The model under review builds one solid part; all positions refer to its coordinate system, in mm. Face numbers are marked on the shaded views. A direction names the side the tool comes from. Give positions to 0.01 mm unless a question says otherwise; leave off trailing zeros. Loops run counter-clockwise (first coordinate to the right, second up) from the corner with the lowest first, then second, coordinate; pieces in that order, holes last. Notation, with made-up numbers: M 14,84 L 33,84 A23 ccw 33,116 Z; hole C 85,25 d10. An arc over 180 degrees is marked long. Return JSON: item names as keys, results as strings.
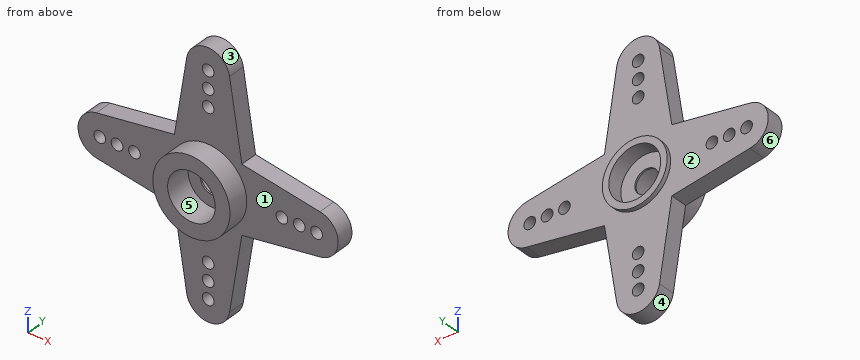
Autodesk Inventor part; units mm, degrees
ref_plane "YZ Plane" through (0, 0, 0) normal (1, 0, 0) x (0, 1, 0)
ref_plane "XZ Plane" through (0, 0, 0) normal (0, 1, 0) x (-1, 0, 0)
ref_plane "XY Plane" through (0, 0, 0) normal (0, 0, 1) x (1, 0, 0)
sketch "Sketch1" plane through (0, 0, 0) normal (0, 1, 0) x (-1, 0, 0)
  circle A0 centre (0, 0) radius 10.5 construction
  circle A1 centre (0, 0) radius 12.5 construction
  circle A2 centre (0, 0) radius 8.5 construction
  circle A3 centre (12.5, 0) radius 2.5
  circle A4 centre (12.5, 0) radius 0.675
  circle A5 centre (10.5, 0) radius 0.675
  circle A6 centre (8.5, 0) radius 0.675
  line L0 (0, 16.4462) -> (0, -19.2601)
  circle A7 centre (0, 12.5) radius 0.675
  circle A8 centre (0, 10.5) radius 0.675
  circle A9 centre (0, 12.5) radius 2.5
  circle A10 centre (0, 8.5) radius 0.675
  circle A11 centre (-12.5, 0) radius 0.675
  circle A12 centre (-10.5, 0) radius 0.675
  circle A13 centre (-12.5, 0) radius 2.5
  circle A14 centre (-8.5, 0) radius 0.675
  circle A15 centre (0, -12.5) radius 0.675
  circle A16 centre (0, -10.5) radius 0.675
  circle A17 centre (0, -12.5) radius 2.5
  circle A18 centre (0, -8.5) radius 0.675
  line L1 (0, 0) -> (7.0711, -7.0711) construction
  line L2 (0, 0) -> (10, 0) construction
  line L3 (0, 0) -> (7.0711, 7.0711) construction
  line L4 (0, 0) -> (10, 0) construction
  line L5 (0, 0) -> (7.0711, -7.0711) construction
  line L6 (0, 0) -> (10, 0) construction
  line L7 (0, 0) -> (-7.0711, -7.0711) construction
  line L8 (0, 0) -> (10, 0) construction
  line L9 (3.8872, -3.8872) -> (12.8889, -2.4696)
  line L10 (3.8872, -3.8872) -> (2.4696, -12.8889)
  line L11 (3.8872, 3.8872) -> (2.4696, 12.8889)
  line L12 (3.8872, 3.8872) -> (12.8889, 2.4696)
  line L13 (-3.8872, 3.8872) -> (-12.8889, 2.4696)
  line L14 (-3.8872, 3.8872) -> (-2.4696, 12.8889)
  line L15 (-3.8872, -3.8872) -> (-2.4696, -12.8889)
  line L16 (-3.8872, -3.8872) -> (-12.8889, -2.4696)
  point P0 (13.5701, 2.2594)
  point P1 (14.0204, -1.9845)
  point P2 (-2.2594, 13.5701)
  point P3 (1.9845, 14.0204)
  point P4 (-13.5701, -2.2594)
  point P5 (-14.0204, 1.9845)
  point P6 (2.2594, -13.5701)
  point P7 (-1.9845, -14.0204)
  dimension "d0" = 21
  dimension "d1" = 25
  dimension "d2" = 17
  dimension "d3" = 5
  dimension "d4" = 1.35
  dimension "d5" = 1.35
  dimension "d6" = 1.35
  dimension "d9" = 360
  dimension "d11" = 10
  dimension "d12" = 45
  dimension "d13" = 10
  dimension "d14" = 45
  dimension "d15" = 10
  dimension "d16" = 45
  dimension "d17" = 10
  dimension "d18" = 135
  dimension "d19" = 107.9
  dimension "d20" = 12.5
  dimension "d21" = 10.5
  dimension "d22" = 2
  dimension "d23" = 8.5
  dimension "d24" = 8.5
  dimension "d25" = 10.5
  dimension "d26" = 12.5
  dimension "d27" = 12.5
  dimension "d30" = 360
extrude "Extrusion1" add sketch "Sketch1" along normal blind 2 contours A3 A5 | A3 A5 L9 L10 A17 A16 L0 A18 A10 A8 A9 L11 L12 | A9 A8 L0 A7 | A17 L0 A15 A16 | L0 A7 A8 A9 | A17 A16 L0 A15 | A9 A8 L0 A10 A18 A16 A17 L15 L16 A13 A12 L13 L14 | A13 A12 picked at (11.2959, 0.9935) picked at (-11.3085, -0.9832)
sketch "Sketch2" plane through (0, 2, 0) normal (0, 1, 0) x (1, 0, 0)
  circle A0 centre (0, 0) radius 3.74
  circle A1 centre (0, 0) radius 2.99
  circle A2 centre (0, 0) radius 1.37
  dimension "d34" = 7.48
  dimension "d35" = 5.98
  dimension "d36" = 2.74
extrude "Extrusion2" add sketch "Sketch2" along normal blind 0.5 contours A0
extrude "Extrusion3" cut sketch "Sketch2" against normal blind 1.25 contours A1
extrude "Extrusion4" cut sketch "Sketch2" against normal through all contours A2
sketch "Sketch3" plane through (0, 0, 0) normal (0, -1, 0) x (1, 0, 0)
  circle A0 centre (0, 0) radius 1.37
  circle A1 centre (0, 0) radius 2.75
  circle A2 centre (0, 0) radius 4.45
  dimension "d43" = 5.5
  dimension "d44" = 8.9
extrude "Extrusion5" add sketch "Sketch3" along normal blind 2.44 contours A2
extrude "Extrusion6" cut sketch "Sketch3" against normal blind 0.56 contours A1
properties part number "MMAE 232 CAD Assignment 2 Servo Horn 5-Nicholas Skiba"
1) Consider section C-C on y = -0.4. Write out the cut boundary in (x, z), then the cut area to 3 significant figures.
From the geometry:
{"outline": "C 0,0 d8.9; hole C 0,0 d5.5", "area": "38.5 mm²"}
2) Consider section D-D on z = 6.75. Write out the cut boundary in (x, y).
From the geometry:
{"outline": "M -3.44,0 L 3.44,0 L 3.44,2 L -3.44,2 Z"}
3) The part is to be moulded in two halves that separate along Z. For the marked faces 4, 5 and 6, say which applies: released by +Z, released by -Z, zero draft, split by the parting line, or undercut.
From the geometry:
{"face 4": "released by -Z", "face 5": "undercut", "face 6": "split by the parting line"}
4) Consider section B-B on z = -10.5. Write out the cut boundary in (x, y) (3 decimals), then the cut area to 3 significant figures.
From the geometry:
{"outline": "M -2.846,0 L -0.675,0 L -0.675,2 L -2.846,2 Z; M 0.675,0 L 2.846,0 L 2.846,2 L 0.675,2 Z", "area": "8.68 mm²"}
5) Tool access review of the marked faces 1, 2 and 3: name each direction out of +Z, -Z, +X, -X, +Y, -Y from which nothing blocks a thin tool from reaching the whole face with its end or side.
From the geometry:
{"face 1": "-Y", "face 2": "+Y", "face 3": "+Z, +Y, -Y"}
6) Insertion check: pin 1 (12 mm diameter, centred on x = -6.5, z = 10.5, fed in from +Y); pin 2 (6 mm diameter, centred on x = 6.5, z = -5.5, fed in from -Y); pin 3 (3 mm diameter, centred on x = 1, z = 0, fed in from +Y). Each pin has a flat end and moves straight along its axis. Give the tip position at first contact, or say it passes through.
From the geometry:
{"pin 1": "y = 2", "pin 2": "y = 0", "pin 3": "y = 0.75"}
7) Consider section A-A on x = -12.5. Write out the cut boundary in (y, z) (3 decimals), then the cut area to 3 significant figures.
From the geometry:
{"outline": "M 0,-2.531 L 2,-2.531 L 2,-0.675 L 0,-0.675 Z; M 0,0.675 L 2,0.675 L 2,2.531 L 0,2.531 Z", "area": "7.42 mm²"}
8) Wall thickness on L1, parallel to Z at x = 0, y = -0.2; L2, parallel to X at y = -0.4, z = -0.5; L3, parallel to Z at x = 12.5, y = 0.95 (3 decimals): over which ranges is each line inside the solid? List them lowest first. Write a range as from..to.
From the geometry:
{"L1": "-4.45..-2.75, 2.75..4.45", "L2": "-4.42..-2.7, 2.7..4.42", "L3": "-2.531..-0.675, 0.675..2.531"}
